Autodesk Inventor part; units mm, degrees
ref_plane "工作平面1" through (0, -10.6214, 5) normal (1, 0, 0) x (0, 0, -1)
ref_plane "YZ Plane" through (0, 0, 0) normal (1, 0, 0) x (0, 1, 0)
ref_plane "XZ Plane" through (0, 0, 0) normal (0, 1, 0) x (-1, 0, 0)
sketch "草图1" plane through (0, 0, 0) normal (0, 0, 1) x (1, 0, 0)
  circle A0 centre (0, 0) radius 4.1
  circle A1 centre (0, 0) radius 7.1
  dimension "d0" = 8.2
  dimension "d1" = 3
extrude "拉伸1" add sketch "草图1" along normal blind 5
sketch "草图2" plane through (0, 0, 5) normal (0, 0, 1) x (1, 0, 0)
  point P0 (0, 0)
sketch "草图3" plane through (0, 0, 5) normal (0, 0, 1) x (1, 0, 0)
  circle A0 centre (0, 0) radius 7.1
  line L0 (-7.1, 0) -> (7.1, 0)
  line L1 (7.1, 0) -> (7.1, -10.6214)
  line L2 (7.1, -10.6214) -> (-7.1, -10.6214)
  line L3 (-7.1, -10.6214) -> (-7.1, 0)
  line L4 (-7.9158, -10.621) -> (28.0842, -10.6393)
  point P0 (7.1, 0)
extrude "拉伸2" add sketch "草图3" against normal blind 5 contours L1 L2 L3 A0
sketch "草图4" plane through (0, 0, 5) normal (0, 0, 1) x (1, 0, 0)
  circle A0 centre (-4.1, -7.6214) radius 1.4
  line L0 (-7.1, -10.6214) -> (7.1, -10.6214)
  line L1 (-7.1, 0) -> (-7.1, -10.6214)
  point P0 (0, 0)
  dimension "d6" = 2.8
  dimension "d7" = 3
  dimension "d8" = 3
extrude "拉伸3" cut sketch "草图4" against normal blind 5
ref_plane "工作平面1" through (0, -10.6214, 5) normal (1, 0, 0) x (0, 0, -1)
mirror "镜像1" about plane through (0, -10.6214, 5) normal (1, 0, 0) of "拉伸3"
properties part number "Z轴"
Design review of the part built by this model. Coordinates are the model's own, in mm. Coordinates: 2 decimals unless noted, no trailing zeros. Order: outer loops, then holes, each group sorted by start corner. A loop starts at its lowest first (then second) coordinate and runs counter-clockwise, first axis right, second up. Notation, with made-up numbers: (22, 64) -> (47, 64) arc R26 cw to (47, 80) -> close; hole circle Ø3 at (30, 55.5). An arc over 180 degrees is marked (long way). Use one line per item in the form item = value. Start each with the question number.
(1) Add section D-D on x = 2.5. State the section outline as (y, z) points, plus the area to 3 significant figures.
(2) Add section B-B on z = 4.65. State the section outline as (x, y) points.
(3) The part is to be moulded in two halves that separate along X. For faces 1 (the cylindrical face through (-0.534, -4.065, 2.465)), 2 (the flat face through (-7.1, -5, 3)), 3 (the flat face through (7.1, -5, 3)), say which applies: +X half, -X half, draft (parallel to the pull), parting line (faces both ways), or undercut.
(4) Add section C-C on x = -3.5. State the section outline as (y, z) points, plus the area to 3 significant figures.
(5) Add section A-A on x = 0. State the section outline as (y, z) points, plus the area to 3 significant figures.
(6) Insertion check: pin 1 (3 mm diameter, centred on x = 1.5, z = 4, fed in from +Y); pin 2 (1.5 mm diameter, centred on x = -4, z = 1, fed in from +Y). Each pin has a flat end and moves straight along its axis. Give the tip position at first contact, or say it passes through.
(7) For probe 1 along X at (y, z) = (-7.5, 2.95); probe 2 along Y at (x, z) = (3.25, 3.45); probe 3 along Y at (x, z) = (3, 2.75), list the stretches that pass through material, from the lowest coordinate up.
Answer block:
q1.outline = (-10.62, 0) -> (-3.25, 0) -> (-3.25, 5) -> (-10.62, 5) -> close; (3.25, 0) -> (6.65, 0) -> (6.65, 5) -> (3.25, 5) -> close
q1.area = 53.8 mm²
q2.outline = (-7.1, -10.62) -> (7.1, -10.62) -> (7.1, 0) arc R7.1 ccw to (-7.1, 0) -> close; hole circle Ø2.8 at (-4.1, -7.62); hole circle Ø8.2 at (0, 0); hole circle Ø2.8 at (4.1, -7.62)
q3.face_1 = undercut
q3.face_2 = -X half
q3.face_3 = +X half
q4.outline = (-10.62, 0) -> (-8.89, 0) -> (-8.89, 5) -> (-10.62, 5) -> close; (-6.36, 0) -> (-2.14, 0) -> (-2.14, 5) -> (-6.36, 5) -> close; (2.14, 0) -> (6.18, 0) -> (6.18, 5) -> (2.14, 5) -> close
q4.area = 50.0 mm²
q5.outline = (-10.62, 0) -> (-4.1, 0) -> (-4.1, 5) -> (-10.62, 5) -> close; (4.1, 0) -> (7.1, 0) -> (7.1, 5) -> (4.1, 5) -> close
q5.area = 47.6 mm²
q6.pin_1 = 7.1
q6.pin_2 = 6.31
q7.probe_1 = -7.1 to -5.49, -2.71 to 2.71, 5.49 to 7.1
q7.probe_2 = -10.62 to -8.73, -6.51 to -2.5, 2.5 to 6.31
q7.probe_3 = -10.62 to -8.49, -6.76 to -2.79, 2.79 to 6.44
